For this review, take the finished solid that the model builds, in its own axes (mm). Face numbers are marked on the shaded views. Round coordinates to 2 decimals unless told otherwise and drop trailing zeros. Loops run counter-clockwise (first coordinate to the right, second up) from the corner with the lowest first, then second, coordinate; pieces in that order, holes last. Notation, with made-up numbers: (-3.75, -24) -> (6.25, -24) arc R28 ccw to (6.25, 1) -> close; hole circle Ø5 at (20.5, -14.75). An arc over 180 degrees is marked (long way). Write each question's results on one line, items separated by ' | '.
```python
from build123d import *

# Parameters (mm, degrees)
F0_R     = 42.676453
F1_DEPTH = 163.83
F2_R     = 42.676453
F2_R_2   = 16.977509
F2_R_3   = 5.550938
F2_W     = 9.032015
F2_H     = 4.260384
F2_W_2   = 9.884089
F2_H_2   = 5.794122
F2_R_4   = 7.978639
F2_W_3   = 9.032009
F2_H_3   = 5.453291
F2_W_4   = 10.395335
F2_H_4   = 6.475783
F2_W_5   = 10.22492
F2_H_5   = 5.623706
F2_W_6   = 9.032014
F2_W_7   = 9.543261
F2_H_6   = 6.98703
F2_W_8   = 10.736168
F2_H_7   = 5.964537
F2_W_9   = 9.884088
F2_H_8   = 5.282876
F2_W_10  = 10.736166
F2_H_9   = 6.987029
F2_W_11  = 8.520767
F2_W_12  = 9.543257
F2_H_10  = 5.282875
F2_H_11  = 6.816613
F3_DEPTH = 25.4


with BuildPart() as f1:
    # F0 (on Top) → F1 (new body)
    with BuildSketch(Plane.XY):
        Circle(F0_R)
    extrude(amount=F1_DEPTH)

    # F2 (on face) → F3 (join)
    with BuildSketch(Plane.XY.offset(163.83)):
        Circle(F2_R)
        with Locations((-4.856836, -21.983579)):
            Circle(F2_R_2, mode=Mode.SUBTRACT)
        with Locations((-30.930383, -14.314889)):
            Circle(F2_R_3, mode=Mode.SUBTRACT)
        with Locations((-31.015591, -0.255623)):
            Rectangle(F2_W, F2_H, mode=Mode.SUBTRACT)
        with Locations((-14.229681, -1.022492)):
            Rectangle(F2_W_2, F2_H_2, mode=Mode.SUBTRACT)
        with Locations((25.477093, -17.211949)):
            Circle(F2_R_4, mode=Mode.SUBTRACT)
        with Locations((34.083065, -0.170416)):
            Rectangle(F2_W_3, F2_H_3, mode=Mode.SUBTRACT)
        with Locations((-30.504344, 9.713674)):
            Rectangle(F2_W_4, F2_H_4, mode=Mode.SUBTRACT)
        with Locations((-7.413067, 9.458051)):
            Rectangle(F2_W_5, F2_H_5, mode=Mode.SUBTRACT)
        with Locations((-19.256933, 18.149234)):
            Rectangle(F2_W_6, F2_H_5, mode=Mode.SUBTRACT)
        with Locations((-13.718434, 27.181246)):
            Rectangle(F2_W_7, F2_H_6, mode=Mode.SUBTRACT)
        with Locations((10.054506, 0.085207)):
            Rectangle(F2_W_8, F2_H_7, mode=Mode.SUBTRACT)
        with Locations((13.718434, 9.969297)):
            Rectangle(F2_W_9, F2_H_8, mode=Mode.SUBTRACT)
        with Locations((3.067476, 17.467572)):
            Rectangle(F2_W_10, F2_H_9, mode=Mode.SUBTRACT)
        with Locations((32.464124, 9.969297)):
            Rectangle(F2_W_11, F2_H_8, mode=Mode.SUBTRACT)
        with Locations((25.817924, 18.319649)):
            Rectangle(F2_W_12, F2_H_10, mode=Mode.SUBTRACT)
        with Locations((9.11722, 27.777701)):
            Rectangle(F2_W_12, F2_H_11, mode=Mode.SUBTRACT)
    extrude(amount=F3_DEPTH)


solid = f1.part
```
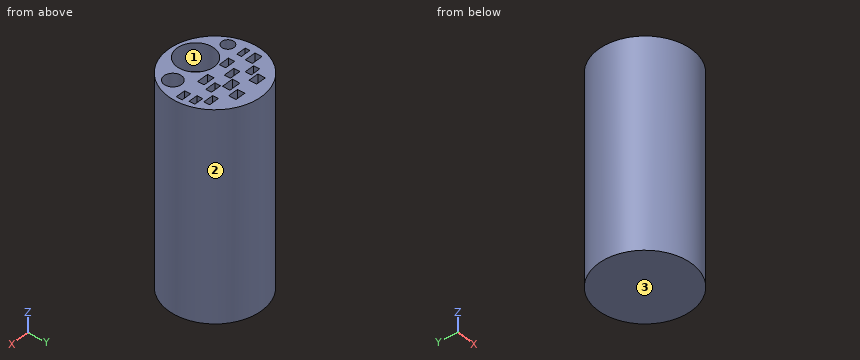
1. Draft analysis for pull direction Y (two halves, no side actions). For the marked faces 1, 2 and 3, state which applies: released by +Y, released by -Y, zero draft, split by the parting line, or undercut.
Values found:
face 1: undercut | face 2: split by the parting line | face 3: zero draft
2. Consider section B-B (z = 47.5). State the section outline as (x, y) points.
Values found:
outline: circle Ø85.35 at (0, 0)
3. Consider section A-A (y = 0). State the section outline as (x, z) points.
Values found:
outline: (-42.68, 0) -> (42.68, 0) -> (42.68, 189.23) -> (38.6, 189.23) -> (38.6, 163.83) -> (29.57, 163.83) -> (29.57, 189.23) -> (15.42, 189.23) -> (15.42, 163.83) -> (4.69, 163.83) -> (4.69, 189.23) -> (-9.29, 189.23) -> (-9.29, 163.83) -> (-19.17, 163.83) -> (-19.17, 189.23) -> (-26.5, 189.23) -> (-26.5, 163.83) -> (-35.53, 163.83) -> (-35.53, 189.23) -> (-42.68, 189.23) -> close
4. Consider section D-D (z = 176). Give the number of separate pieces and of enclosed holes in the cut face, plus the area to 3 significant figures.
Values found:
separate pieces: 1 | enclosed holes: 16 | area: 3,780 mm2
5. To check wall thickness, follow probe 1 along X at (y, z) = (-13.5, 174.5); probe 2 along Y at (x, z) = (-27.5, 182); probe 3 along Y at (x, z) = (-3.5, 181.5). State the ranges of each line that lie inside material, in increasing order.
Values found:
probe 1: x = -40.48 to -36.42, -25.44 to -19.56, 9.85 to 18.41, 32.54 to 40.48 | probe 2: y = -32.63 to -18.68, -9.95 to -2.39, 1.87 to 6.48, 12.95 to 32.63 | probe 3: y = -42.53 to -38.91, -5.06 to 6.65, 12.27 to 42.53
6. For pin 1 (10 mm diameter, centred on x = -2.5, z = 122.5, fed in from -Y); pin 2 (1.5 mm diameter, centred on y = 15.5, z = 110.5, fed in from +X); pin 3 (4.5 mm diameter, centred on x = -19, z = 180, fed in from +Y), all flat-tipped, find the tip position at first contact; note any pin that passes through.
Values found:
pin 1: stops at y = -42.68 | pin 2: stops at x = 40.05 | pin 3: stops at y = 39.25
7. Consider section C-C (x = 0). State the section outline as (y, z) points.
Values found:
outline: (-42.68, 0) -> (42.68, 0) -> (42.68, 189.23) -> (20.96, 189.23) -> (20.96, 163.83) -> (13.97, 163.83) -> (13.97, 189.23) -> (-5.72, 189.23) -> (-5.72, 163.83) -> (-38.25, 163.83) -> (-38.25, 189.23) -> (-42.68, 189.23) -> close
